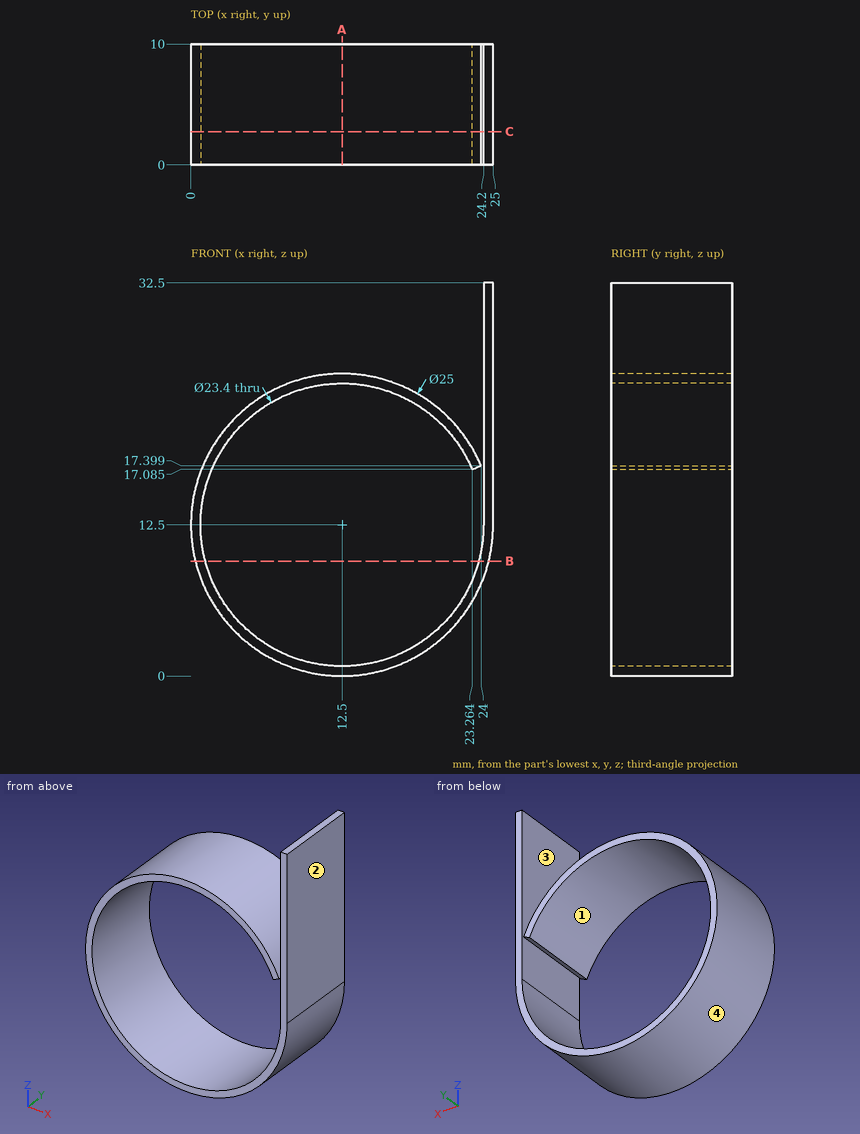
Geometry check sheet. Reference: drawing and pictorial views, mm from the part's lowest x, y, z. A direction names the side the tool comes from. Give positions to 0.01 mm unless a question says otherwise; leave off trailing zeros. Write each loop counter-clockwise with the first axis right and the second up, starting at its lowest first coordinate (ties: lowest second). Pieces come first, ordered by that corner, then holes.
Item 1: Gauge pin test, flat ends, axial feed: pin 1 (2 mm diameter, centred on x = 15.5, z = 27.5, fed in from +Y); pin 2 (4 mm diameter, centred on x = 21.5, z = 6, fed in from -Y); pin 3 (6 mm diameter, centred on x = 21, y = 6.5, fed in from +Z) (1 decimal); pin 4 (5 mm diameter, centred on y = 3, z = 23.5, fed in from -X) (1 decimal). Record the tip position at first contact, or that the pin passes through.
Item 2: Draft check along X on the marked faces 1 and 2. Enter one of: released by +X, released by -X, zero draft, split by the parting line, or undercut.
Item 3: Scan lines: L1, parallel to Z at x = 12.5, y = 4.5; L2, parallel to X at y = 5.5, z = 17.5 (1 decimal). Record each from-to range of solid material in increasing order.
Item 4: Cross-section at A-A (x = 12.5). Enter the section's corners in (y, z), and give its area (3 significant figures).
Item 5: Cross-section at B-B (z = 9.5). Enter the section's corners in (x, y) (1 decimal).
Item 6: Cross-section at C-C (y = 2.75). Enter the section's corners in (x, z) (1 decimal).
Item 7: Access from +Z, -Z, +X, -X, +Y, -Y to the whole of each face (thin tool, end or side, straight path). Record for the marked faces 3 and 4.
Report:
1. pin 1: passes through
1. pin 2: stops at y = 0
1. pin 3: stops at z = 23.7
1. pin 4: stops at x = 3.3
2. face 1: undercut
2. face 2: released by +X
3. L1: z = 0 to 0.8, 24.2 to 25
3. L2: x = 1 to 1.9, 23.1 to 24, 24.2 to 25
4. outline: (0, 0) - (10, 0) - (10, 0.8) - (0, 0.8) - close; (0, 24.2) - (10, 24.2) - (10, 25) - (0, 25) - close
4. area: 16.0 mm2
5. outline: (0.4, 0) - (1.2, 0) - (1.2, 10) - (0.4, 10) - close; (23.8, 0) - (24.6, 0) - (24.6, 10) - (23.8, 10) - close
6. outline: (23.3, 17.1) - (24, 17.4) arc R12.5 ccw (long way) to (25, 12.5) - (25, 32.5) - (24.2, 32.5) - (24.2, 12.5) arc R11.7 cw (long way) to start
7. face 3: +Z, +Y, -Y
7. face 4: +Y, -Y
